Geometry: final body of the model. Coordinates: model frame, mm. Face numbers are marked on the shaded views. Give positions to 0.01 mm unless a question says otherwise; leave off trailing zeros. Write each loop counter-clockwise with the first axis right and the second up, starting at its lowest first coordinate (ties: lowest second). Pieces come first, ordered by that corner, then holes. Notation, with made-up numbers: (33.25, 4.25) - (85.25, 4.25) arc R19 cw to (85.25, 40.25) - close; hole circle Ø6 at (87.5, -10). An arc over 180 degrees is marked (long way). Return JSON: item names as keys, results as strings.
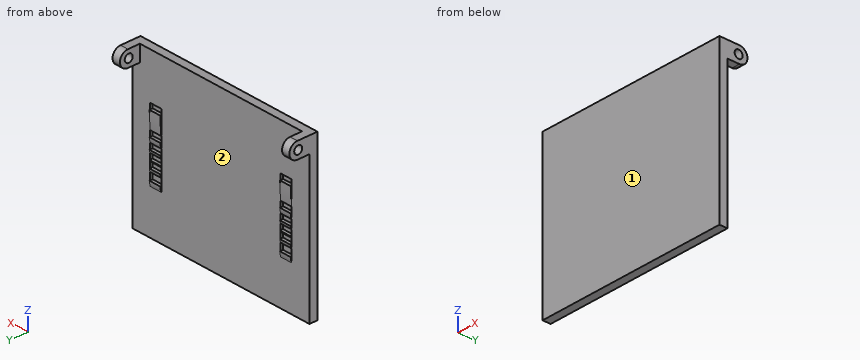
from build123d import *

# Parameters (mm, degrees)
SKETCH1_W           = 304.8
SKETCH1_H           = 254
BOSS_EXTRUDE1_DEPTH = 12.7
SKETCH2_W           = 12.7
SKETCH2_H           = 25.4
BOSS_EXTRUDE2_DEPTH = 19.05
BOSS_EXTRUDE3_DEPTH = 12.7
SKETCH5_R           = 6.35
CUT_EXTRUDE1_DEPTH  = 12.7
SKETCH6_W           = 19.05
SKETCH6_H           = 8.89
SKETCH6_H_2         = 11.176
CUT_EXTRUDE2_DEPTH  = 3.81
BOSS_EXTRUDE4_DEPTH = 19.05


with BuildPart() as part:
    # Sketch1 → Boss-Extrude1 (new body)
    with BuildSketch(Plane(origin=(0, 0, 0), x_dir=(1, 0, 0), z_dir=(0, 1, 0))):
        Rectangle(SKETCH1_W, SKETCH1_H)
    extrude(amount=BOSS_EXTRUDE1_DEPTH)

    # Sketch2 → Boss-Extrude2 (add)
    with BuildSketch(Plane(origin=(0, 12.7, 0), x_dir=(1, 0, 0), z_dir=(0, 1, 0))):
        with Locations((-146.05, -114.3)):
            Rectangle(SKETCH2_W, SKETCH2_H)
    boss_extrude2 = extrude(amount=BOSS_EXTRUDE2_DEPTH)

    # Sketch4 → Boss-Extrude3 (add)
    with BuildSketch(Plane(origin=(-139.7, 0, 0), x_dir=(0, 0, -1), z_dir=(1, 0, 0))):
        with BuildLine():
            Line((-127, 31.75), (-101.6, 31.75))
            ThreePointArc((-101.6, 31.75), (-114.3, 44.45), (-127, 31.75))
        make_face()
    boss_extrude3 = extrude(amount=-BOSS_EXTRUDE3_DEPTH)

    # Sketch5 → Cut-Extrude1 (cut)
    with BuildSketch(Plane(origin=(-139.7, 0, 0), x_dir=(0, 0, -1), z_dir=(1, 0, 0))):
        with Locations((-114.3, 30.48)):
            Circle(SKETCH5_R)
    cut_extrude1 = extrude(amount=-CUT_EXTRUDE1_DEPTH, mode=Mode.SUBTRACT)

    # Mirror1: Boss-Extrude2, Boss-Extrude3, Cut-Extrude1 across plane
    add(boss_extrude2.mirror(Plane(origin=(0, 0, 0), x_dir=(0, 0, 1), z_dir=(1, 0, 0))))
    add(boss_extrude3.mirror(Plane(origin=(0, 0, 0), x_dir=(0, 0, 1), z_dir=(1, 0, 0))))
    add(cut_extrude1.mirror(Plane(origin=(0, 0, 0), x_dir=(0, 0, 1), z_dir=(1, 0, 0))), mode=Mode.SUBTRACT)

    # Sketch6 → Cut-Extrude2 (cut)
    with BuildSketch(Plane(origin=(0, 12.7, 0), x_dir=(1, 0, 0), z_dir=(0, 1, 0))):
        with Locations((-112.395, -50.419)):
            Rectangle(SKETCH6_W, SKETCH6_H)
        with Locations((-112.395, -13.589)):
            Rectangle(SKETCH6_W, SKETCH6_H)
        with Locations((-112.395, 17.145)):
            Rectangle(SKETCH6_W, SKETCH6_H)
        with Locations((-112.395, 3.429)):
            Rectangle(SKETCH6_W, SKETCH6_H)
        with Locations((-112.395, 28.575)):
            Rectangle(SKETCH6_W, SKETCH6_H)
        with Locations((-112.395, 43.942)):
            Rectangle(SKETCH6_W, SKETCH6_H_2)
    cut_extrude2 = extrude(amount=-CUT_EXTRUDE2_DEPTH, mode=Mode.SUBTRACT)

    # Sketch7 → Boss-Extrude4 (add)
    with BuildSketch(Plane.ZY.offset(102.87)):
        with BuildLine():
            Line((45.974, 12.7), (45.974, 13.97))
            ThreePointArc((45.974, 13.97), (31.989575629, 13.652336171), (18.034, 12.7))
            Line((18.034, 12.7), (45.974, 12.7))
        make_face()
        with BuildLine():
            Line((9.144, 12.7), (9.144, 13.97))
            ThreePointArc((9.144, 13.97), (5.030689776, 13.650585434), (1.016, 12.7))
            Line((1.016, 12.7), (9.144, 12.7))
        make_face()
        with BuildLine():
            Line((-7.874, 12.7), (-12.7, 12.7))
            ThreePointArc((-12.7, 12.7), (-10.369154103, 13.647185593), (-7.874, 13.97))
            Line((-7.874, 13.97), (-7.874, 12.7))
        make_face()
        with BuildLine():
            Line((-21.59, 12.7), (-24.13, 12.7))
            ThreePointArc((-24.13, 12.7), (-23.009903166, 13.634806331), (-21.59, 13.97))
            Line((-21.59, 13.97), (-21.59, 12.7))
        make_face()
        with BuildLine():
            Line((-33.02, 12.7), (-38.354, 12.7))
            ThreePointArc((-38.354, 12.7), (-35.761553209, 13.64812348), (-33.02, 13.97))
            Line((-33.02, 13.97), (-33.02, 12.7))
        make_face()
        with BuildLine():
            Line((-49.53, 12.7), (-57.658, 12.7))
            ThreePointArc((-57.658, 12.7), (-53.643310224, 13.650585434), (-49.53, 13.97))
            Line((-49.53, 13.97), (-49.53, 12.7))
        make_face()
    boss_extrude4 = extrude(amount=BOSS_EXTRUDE4_DEPTH)

    # Mirror2: Cut-Extrude2, Boss-Extrude4 across plane
    add(cut_extrude2.mirror(Plane(origin=(0, 0, 0), x_dir=(0, 0, 1), z_dir=(1, 0, 0))), mode=Mode.SUBTRACT)
    add(boss_extrude4.mirror(Plane(origin=(0, 0, 0), x_dir=(0, 0, 1), z_dir=(1, 0, 0))))


solid = part.part
Q1. Section query B-B, the plane x = 58. Return the cut outline in (y, z).
Answer key:
{"outline": "(0, -127) - (12.7, -127) - (12.7, 127) - (0, 127) - close"}
Q2. Material intervals for probe 1 along Y at (x, z) = (143.75, 114.3); probe 2 along Z at (x, y) = (-142, 30); probe 3 along Y at (x, z) = (-8, -93), sorted ascending. Write a range as [from, to].
Answer key:
{"probe 1": "y = [0, 24.13], [36.83, 44.45]", "probe 2": "z = [101.6, 107.97], [120.63, 127]", "probe 3": "y = [0, 12.7]"}
Q3. Pin query (flat end, axial travel): P1, Ø12, axis at x = -10.5, y = 23.5, coming from the +Z side; P2, Ø4.5, axis at x = -113.5, z = -4, coming from the +Y side; P3, Ø12, axis at x = -13.5, z = 38.5, coming from the +Y side; P4, Ø1.4, axis at y = 13.5, z = -35.5, coming from the +X side. Return the tip coordinate at first contact, or that it passes through.
Answer key:
{"P1": "passes through", "P2": "stops at y = 8.89", "P3": "stops at y = 12.7", "P4": "stops at x = 121.92"}
Q4. Section query A-A, the plane z = 114.3. Return the cut outline in (x, y), plus the area to 3 significant figures.
Answer key:
{"outline": "(-152.4, 0) - (152.4, 0) - (152.4, 24.13) - (139.7, 24.13) - (139.7, 12.7) - (-139.7, 12.7) - (-139.7, 24.13) - (-152.4, 24.13) - close; (-152.4, 36.83) - (-139.7, 36.83) - (-139.7, 44.45) - (-152.4, 44.45) - close; (139.7, 36.83) - (152.4, 36.83) - (152.4, 44.45) - (139.7, 44.45) - close", "area": "4,350 mm^2"}
Q5. Mould query, pull axis X, two halves, no side actions, for the marked faces 1 and 2. Classes: pulls with the +X half, pulls with the -X half, needs draft (parallel to the pull), parting line crosses it, or undercut.
Answer key:
{"face 1": "needs draft", "face 2": "undercut"}
